```python
from build123d import *

# Parameters (mm, degrees)
F0_W     = 150
F0_H     = 150
F1_DEPTH = 6


with BuildPart() as f1:
    # F0 (on Top) → F1 (new body)
    with BuildSketch(Plane.XY):
        Rectangle(F0_W, F0_H)
        with BuildLine():
            ThreePointArc((5.7307365463, 18.1151499756), (0, -19), (-5.7307365463, 18.1151499756))
            add(Edge.make_bspline(
                [(5.7307365463, 18.1151499756), (6.2063982555, 30.545456659), (0, 30.545456659), (-6.2063982555, 30.545456659), (-5.7307365463, 18.1151499756)],
                knots=[4.6356732139, 4.6356732139, 4.6356732139, 6.2831853072, 6.2831853072, 7.9306974004, 7.9306974004, 7.9306974004], degree=2, weights=[1, 0.6794701836, 1, 0.6794701836, 1]))
        make_face(mode=Mode.SUBTRACT)
    extrude(amount=F1_DEPTH)


solid = f1.part
```
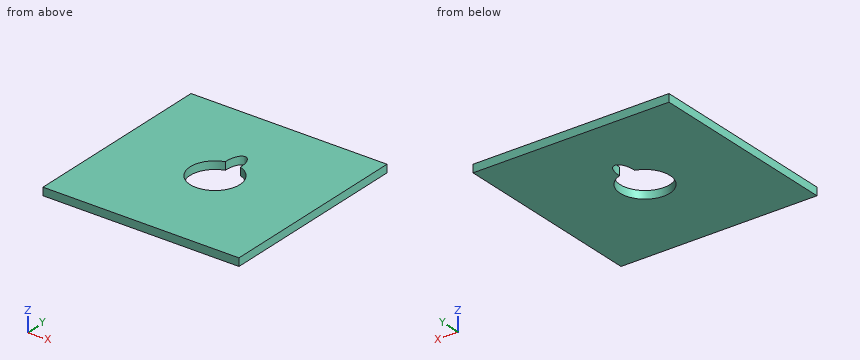
Model file for the job. Use its own axes, mm. Give positions to 0.01 mm unless a question says otherwise; leave off trailing zeros. Write each loop counter-clockwise with the first axis right and the second up, starting at its lowest first coordinate (ties: lowest second). Pieces come first, ordered by that corner, then holes. Notation, with made-up numbers: (-14.75, -4) - (11.25, -4) arc R18 cw to (11.25, 20) - close; hole circle Ø3 at (-31, -38). An arc over 180 degrees is marked (long way). One line per question, with ' | ' between items. Start each with the question number.
(1) Slice it at B-B on x = 16. Write the cut outline in (y, z), plus the area to 3 significant figures.
(2) Wall check: line 1 along X through (y, z) = (0, 1.8); line 2 along Y through (x, z) = (0, 3.45); line 3 along Y through (x, z) = (14, 5.5). Give the ranges that are in metal, low to high. Write a range as from..to.
(3) Slice it at A-A on y = 0. Write the cut outline in (x, z), plus the area to 3 significant figures.
Results below:
1) outline: (-75, 0) - (-10.25, 0) - (-10.25, 6) - (-75, 6) - close; (10.25, 0) - (75, 0) - (75, 6) - (10.25, 6) - close | area: 777 mm^2
2) line 1: -75..-19, 19..75 | line 2: -75..-19, 30.55..75 | line 3: -75..-12.85, 12.85..75
3) outline: (-75, 0) - (-19, 0) - (-19, 6) - (-75, 6) - close; (19, 0) - (75, 0) - (75, 6) - (19, 6) - close | area: 672 mm^2
